Can you work these out from the model? Positions are in its coordinate system, mm. A direction names the side the tool comes from. Coordinates: 2 decimals unless noted, no trailing zeros. Write each loop counter-clockwise with the first axis right and the second up, starting at its lowest first coordinate (ties: lowest second). Pieces come first, ordered by that corner, then holes. Notation, with made-up numbers: (-22.5, 51.5) -> (17.5, 51.5) arc R14 ccw to (17.5, 74.5) -> close; hole circle Ø6 at (88.5, 24.25). An arc over 180 degrees is marked (long way). Use one line per item in the form item = value.
Autodesk Inventor part; units mm, degrees
ref_plane "YZ Plane" through (0, 0, 0) normal (1, 0, 0) x (0, 1, 0)
ref_plane "XZ Plane" through (0, 0, 0) normal (0, 1, 0) x (-1, 0, 0)
ref_plane "XY Plane" through (0, 0, 0) normal (0, 0, 1) x (1, 0, 0)
sketch "Sketch1" plane through (0, 0, 0) normal (0, 0, 1) x (1, 0, 0)
  circle A0 centre (0, 0) radius 50.8
  circle A1 centre (0, 0) radius 31.75
  dimension "d0" = 101.6
  dimension "d1" = 63.5
extrude "Extrusion2" add sketch "Sketch1" along normal blind 25.4 contours A0 | A1
sketch "Sketch4" plane through (0, 0, 0) normal (0, 0, -1) x (-1, 0, 0)
  point P0 (0, 0)
  point P1 (0, 31.75)
  point P2 (-30.196, 9.8113)
  point P3 (0, 0)
  point P4 (-18.6622, -25.6863)
  point P5 (0, 0)
  point P6 (18.6622, -25.6863)
  point P7 (0, 0)
  point P8 (30.196, 9.8113)
  point P9 (0, 0)
  dimension "d12" = 31.75
  dimension "d15" = 360
hole "Hole1" at (0, 31.75, 0) direction (0, 0, 1) diameter 6.35 end through all
hole "Hole2" at (-30.196, 9.8113, 0) at (-18.6622, -25.6863, 0) direction (0, 0, 1) diameter 9.525 end through all counterbore diameter 19.05 counterbore depth 6.35
hole "Hole3" at (18.6622, -25.6863, 0) direction (0, 0, 1) diameter 4.9784 depth 19.05
hole "Hole4" at (30.196, 9.8113, 0) direction (0, 0, 1) diameter 13.4874 depth 19.05
equation "\"d22\" = d12"
equation "\"d29\" = d12"
properties part number "ArthurW5.5aHoles"
Q1. Will these pins go through, and if not, where does the flat tip stop? pin 1 (1 mm diameter, centred on y = 9.5, z = 5, fed in from -X); pin 2 (2 mm diameter, centred on y = 14.5, z = 19, fed in from +X); pin 3 (21 mm diameter, centred on x = -22.5, y = -30.5, fed in from -Z); pin 4 (2.5 mm diameter, centred on x = 19.5, y = -25, fed in from -Z).
Return value:
pin_1 = -50
pin_2 = 48.97
pin_3 = 0
pin_4 = 19.05
Q2. Suppose I cut it at B-B (y = 31.75). Write out the boundary of the cut face in (x, z) (3 decimals).
Return value:
outline = (-39.656, 0) -> (-3.175, 0) -> (-3.175, 25.4) -> (-39.656, 25.4) -> close; (3.175, 0) -> (39.656, 0) -> (39.656, 25.4) -> (3.175, 25.4) -> close
Q3. Suppose I cut it at C-C (z = 3). Write out the boundary of the cut face in (x, y) (3 decimals), then the cut area to 3 significant figures.
Return value:
outline = circle Ø101.6 at (0, 0); hole circle Ø19.05 at (-30.196, 9.811); hole circle Ø19.05 at (-18.662, -25.686); hole circle Ø6.35 at (0, 31.75); hole circle Ø4.978 at (18.662, -25.686); hole circle Ø13.487 at (30.196, 9.811)
area = 7,340 mm2
Q4. Thinking about a two-plate mould opening in X: for faces 3 (the cylindrical face through (-11.012, 49.592, 12.522)), 4 (the flat face through (-20.9, -30.1, 6.35)), 5 (the flat face through (-1, 1, 0)), which applies, released by +X, released by -X, zero draft, split by the parting line, or undercut?
Return value:
face_3 = split by the parting line
face_4 = undercut
face_5 = zero draft
Q5. Suppose I cut it at A-A (x = 0). Write out the boundary of the cut face in (y, z) (3 decimals).
Return value:
outline = (-50.8, 0) -> (28.575, 0) -> (28.575, 25.4) -> (-50.8, 25.4) -> close; (34.925, 0) -> (50.8, 0) -> (50.8, 25.4) -> (34.925, 25.4) -> close
Q6. For faces 1 (the flat face through (19, -26, 19.05)), 2 (the cylindrical face through (-0.14, 28.58, 12.88)), which set-ups out of +Z, -Z, +X, -X, +Y, -Y let a thin tool reach every point of the face, with its end or its side?
Return value:
face_1 = -Z
face_2 = +Z, -Z
Q7. Suppose I cut it at D-D (z = 23.25). Give the number of separate pieces and of enclosed holes in the cut face, then the cut area to 3 significant figures.
Return value:
separate_pieces = 1
enclosed_holes = 3
area = 7,930 mm2
Q8. If I drill on line 1 (Y direction, x = 0, z = 10.25) (3 decimals); line 2 (X direction, y = 4.5, z = 16.5); line 3 (Z direction, x = -22.5, y = -21), over which ranges is the centre line in solid material (lowest first)? Write a range as from..to.
Return value:
line_1 = -50.8..28.575, 34.925..50.8
line_2 = -50.6..26.04, 34.35..50.6
line_3 = 6.35..25.4
